Verification items for the finished model (mm, model axes). Face numbers are marked on the shaded views. A direction names the side the tool comes from. Round coordinates to 2 decimals unless told otherwise and drop trailing zeros. Write each loop counter-clockwise with the first axis right and the second up, starting at its lowest first coordinate (ties: lowest second). Pieces come first, ordered by that corner, then holes. Notation, with made-up numbers: (6, 69) - (10, 69) arc R16 cw to (10, 87) - close; hole circle Ø1 at (88, 2.5). An arc over 180 degrees is marked (long way). Write each question's results on one line, items separated by ' | '.
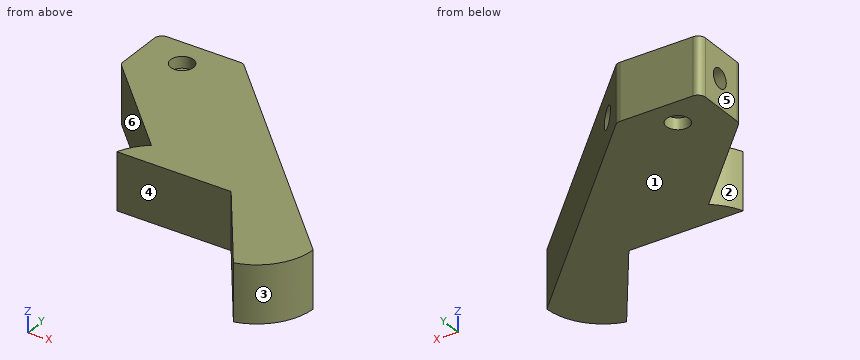
Autodesk Inventor part; units mm, degrees
ref_plane "YZ Plane" through (0, 0, 0) normal (1, 0, 0) x (0, 1, 0)
ref_plane "XZ Plane" through (0, 0, 0) normal (0, 1, 0) x (-1, 0, 0)
ref_plane "XY Plane" through (0, 0, 0) normal (0, 0, 1) x (1, 0, 0)
sketch "Sketch1" plane through (0, 0, 0) normal (0, 0, 1) x (1, 0, 0)
  line L0 (0, 0) -> (0, 15)
  line L1 (0, 15) -> (22, 15)
  line L2 (22, 15) -> (78.5685, -41.5685)
  line L3 (0, 0) -> (24.7487, -24.7487)
  line L4 (0, 0) -> (35, 0) construction
  line L5 (0, 15) -> (0, 7.5) construction
  line L6 (11.1378, 7.6884) -> (50.0287, -31.2025) construction
  line L7 (11.1378, 7.6884) -> (66.1378, 7.6884) construction
  line L8 (50.0287, -31.2025) -> (67.2359, -55.777)
  line L9 (50.0287, -31.2025) -> (80.0287, -31.2025) construction
  line L10 (50.0287, -31.2025) -> (20.0287, -31.2025)
  arc A0 (24.7487, -24.7487) -> (20.0287, -31.2025) centre (34.0582, -36.5103) ccw
  arc A1 (67.2359, -55.777) -> (78.5685, -41.5685) centre (63.5723, -41.2313) ccw
  dimension "d0" = 15
  dimension "d1" = 22
  dimension "d2" = 80
  dimension "d3" = 135
  dimension "d4" = 35
  dimension "d5" = 45
  dimension "d6" = 55
  dimension "d7" = 45
  dimension "d8" = 30
  dimension "d9" = 55
  dimension "d10" = 30
  dimension "d11" = 15
  dimension "d12" = 15
extrude "Extrusion1" add sketch "Sketch1" along normal blind 15
sketch "Sketch2" plane through (0, 0, 0) normal (-1, 0, 0) x (0, 0, 1)
  line L0 (0, -41.5685) -> (0, 15) construction
  line L1 (0, 15) -> (7.5, 15) construction
  line L2 (0, 15) -> (15, 15) construction
  line L3 (7.5, 15) -> (7.5, 7.5) construction
  circle A0 centre (7.5, 7.5) radius 2.5
  point P0 (0, 0)
  dimension "d15" = 7.5
  dimension "d16" = 7.5
  dimension "d17" = 5
extrude "Extrusion2" cut sketch "Sketch2" against normal blind 33
fillet "Fillet1" radius 2 2 edges at (0, 15, 7.5) (0, 0, 7.5)
fillet "Fillet2" radius 2 1 edges at (22, 15, 7.5)
sketch "Sketch3" plane through (0, 0, 15) normal (0, 0, 1) x (1, 0, 0)
  line L0 (21.1716, 15) -> (2, 15) construction
  line L1 (6.35, 15) -> (6.35, 7.5) construction
  line L2 (0, 13) -> (0, 0.8284) construction
  line L3 (0, 7.5) -> (11, 7.5) construction
  line L4 (0, 7.5) -> (11, 7.5) construction
  circle A0 centre (11, 7.5) radius 3
  point P0 (0, 0)
  dimension "d22" = 7.5
  dimension "d23" = 11
  dimension "d24" = 0
  dimension "d25" = 6
extrude "Extrusion3" cut sketch "Sketch3" against normal blind 3
sketch "Sketch4" plane through (0, 0, 0) normal (0, 0, -1) x (-1, 0, 0)
  line L0 (-21.1716, 15) -> (-2, 15) construction
  line L1 (-4.7625, 15) -> (-4.7625, 7.5) construction
  line L2 (-4.7625, 15) -> (2.7375, 15) construction
  line L3 (0, 13) -> (0, 0.8284) construction
  line L4 (0, 7.5) -> (-11, 7.5) construction
  line L5 (0, 7.5) -> (11, 7.5) construction
  circle A0 centre (-11, 7.5) radius 3
  point P0 (0, 0)
  dimension "d28" = 7.5
  dimension "d29" = 90
  dimension "d30" = 11
  dimension "d31" = 180
  dimension "d32" = 6
extrude "Extrusion4" cut sketch "Sketch4" against normal blind 3
properties part number "Ramię ze szczękami" material "Steel"
(1) Thickness scan on L1, parallel to Z at x = 22, y = 7.5; L2, parallel to Y at x = 26.5, z = 12.25; L3, parallel to Y at x = 11, z = 2.2. Record the ranges inside material, lowest first.
Answer:
L1: 0 to 5, 10 to 15 | L2: -31.2 to 10.5 | L3: -11 to 4.5, 10.5 to 15
(2) Section check A-A (z = 7.5). Record the cut outline in (x, y), plus the area to 3 significant figures.
Answer:
outline: (0, 0.83) arc R2 ccw to (0.59, -0.59) - (24.75, -24.75) arc R15 ccw to (20.03, -31.2) - (50.03, -31.2) - (67.24, -55.78) arc R15 ccw to (78.57, -41.57) - (32, 5) - (0, 5) - close; (0, 10) - (27, 10) - (22.59, 14.41) arc R2 ccw to (21.17, 15) - (2, 15) arc R2 ccw to (0, 13) - close | area: 1,880 mm2
(3) Mould release check, pull along Y, two halves, no side actions. Record for the marked faces 1, 2 and 3: released by +Y, released by -Y, zero draft, split by the parting line, or undercut.
Answer:
face 1: zero draft | face 2: undercut | face 3: released by -Y
(4) Section check C-C (x = 11). Record the cut outline in (y, z).
Answer:
outline: (-11, 0) - (4.5, 0) - (4.5, 3) - (10.5, 3) - (10.5, 0) - (15, 0) - (15, 15) - (10.5, 15) - (10.5, 12) - (4.5, 12) - (4.5, 15) - (-11, 15) - close; hole circle Ø5 at (7.5, 7.5)
(5) Go/stop test with flat-tipped pins: pin 1 Ø5.5 at (x, y) = (11, 7.5) entering from -Z; pin 2 Ø1.8 at (x, y) = (9.5, 8) entering from +Z; pin 3 Ø1 at (y, z) = (-27.5, 8) entering from -X. Record where each tip stops, or that it passes through.
Answer:
pin 1: z = 3 | pin 2: z = 12 | pin 3: x = 21.71
(6) Section check D-D (y = -15). Record the cut outline in (x, z), plus the area to 3 significant figures.
Answer:
outline: (15, 0) - (52, 0) - (52, 15) - (15, 15) - close | area: 555 mm2
(7) Set-up check for the marked faces 4, 5 and 6: record each of +Z, -Z, +X, -X, +Y, -Y from which the full face is reachable in a straight line by a thin tool's end or side.
Answer:
face 4: +Z, -Z, -X, -Y | face 5: +Z, -Z, -X, +Y, -Y | face 6: +Z, -Z, -X
(8) Section check B-B (y = 7.5). Record the cut outline in (x, z), plus the area to 3 significant figures.
Answer:
outline: (0, 0) - (8, 0) - (8, 3) - (14, 3) - (14, 0) - (29.5, 0) - (29.5, 5) - (0, 5) - close; (0, 10) - (29.5, 10) - (29.5, 15) - (14, 15) - (14, 12) - (8, 12) - (8, 15) - (0, 15) - close | area: 259 mm2
